Autodesk Inventor part; units mm, degrees
ref_plane "YZ Plane" through (0, 0, 0) normal (1, 0, 0) x (0, 1, 0)
ref_plane "XZ Plane" through (0, 0, 0) normal (0, 1, 0) x (-1, 0, 0)
ref_plane "XY Plane" through (0, 0, 0) normal (0, 0, 1) x (1, 0, 0)
sketch "Sketch1" plane through (0, 0, 0) normal (0, 0, 1) x (1, 0, 0)
  line L0 (0, 0) -> (60.5112, 0)
  line L1 (60.5112, 0) -> (60.5112, -41.275)
  line L2 (60.5112, -41.275) -> (0, -41.275)
  line L3 (0, -41.275) -> (0, 0)
  dimension "d0" = 41.275
  dimension "d1" = 60.5112
extrude "Extrusion1" add sketch "Sketch1" against normal blind 1.5875
sketch "Sketch2" plane through (0, 0, 0) normal (0, 0, 1) x (1, 0, 0)
  line L0 (0, 0) -> (60.5112, 0)
  line L1 (0, -41.275) -> (0, 0)
  line L2 (60.5112, -41.275) -> (0, -41.275)
  line L3 (60.5112, 0) -> (60.5112, -41.275)
  circle A0 centre (2.8067, -33.7185) radius 1.5875
  circle A1 centre (57.7045, -33.7185) radius 1.5875
  circle A2 centre (9.4234, -2.8067) radius 1.5875
  circle A3 centre (51.0878, -2.8067) radius 1.5875
  dimension "d13" = 3.175
  dimension "d14" = 2.8067
  dimension "d15" = 7.5565
  dimension "d16" = 3.175
  dimension "d17" = 7.5565
  dimension "d18" = 2.8067
  dimension "d19" = 3.175
  dimension "d20" = 9.4234
  dimension "d21" = 9.4234
  dimension "d22" = 3.175
  dimension "d23" = 2.8067
  dimension "d24" = 2.8067
extrude "Extrusion2" cut sketch "Sketch2" against normal blind 1.5875 contours A0 | A1 | A2 | A3
properties part number "Sensor Case Lid"
Geometry check sheet. Reference: the model listing, model coordinates, mm. Round coordinates to 2 decimals unless told otherwise and drop trailing zeros. Order: outer loops, then holes, each group sorted by start corner. A loop starts at its lowest first (then second) coordinate and runs counter-clockwise, first axis right, second up. Notation, with made-up numbers: M 41,-28.75 L 58,-28.75 A14 cw 58,-18.75 Z; hole C 25,36 d2. An arc over 180 degrees is marked long. Answer in a Markdown table with one row per item.
(1) Scan lines: probe 1 along X at (y, z) = (-33.5, -0.95); probe 2 along X at (y, z) = (-33, -0.45); probe 3 along Y at (x, z) = (9.5, -0.35) (3 decimals). Record each from-to range of solid material in increasing order. Write a range as from..to.
Responses:
| item | result |
|---|---|
| probe 1 | x = 0..1.23, 4.38..56.13, 59.28..60.51 |
| probe 2 | x = 0..1.39, 4.22..56.29, 59.12..60.51 |
| probe 3 | y = -41.275..-4.392, -1.221..0 |
(2) Sectioned sample at A-A, the plane x = 51. Record the cut outline in (y, z) (1 decimal), and give its area (3 significant figures).
Responses:
| item | result |
|---|---|
| outline | M -41.3,-1.6 L -4.4,-1.6 L -4.4,0 L -41.3,0 Z; M -1.2,-1.6 L 0,-1.6 L 0,0 L -1.2,0 Z |
| area | 60.5 mm² |
(3) Draft check along X on faces 1 (the face through (0, -21, -1)), 2 (the face through (58.437, -35.127, -0.783)), 3 (the face through (30, -20, -1.588)), 4 (the face through (60.511, -20, -1)). Enter one of: released by +X, released by -X, zero draft, split by the parting line, or undercut.
Responses:
| item | result |
|---|---|
| face 1 | released by -X |
| face 2 | undercut |
| face 3 | zero draft |
| face 4 | released by +X |
